from build123d import *

# Parameters (mm, degrees)
F0_W     = 12.7
F0_H     = 12.7
F0_R     = 2.54
F1_DEPTH = 6.35
F2_SIZE  = 2.54
F3_R     = 0.254


with BuildPart() as f1:
    # F0 (on Top) → F1 (new body)
    with BuildSketch(Plane.XY):
        Rectangle(F0_W, F0_H)
        Circle(F0_R, mode=Mode.SUBTRACT)
    extrude(amount=F1_DEPTH)

    # F2
    f2_edges = [f1.edges().sort_by_distance(p)[0] for p in [
        (-2.54, 0, 0),
    ]]
    chamfer(f2_edges, length=F2_SIZE)

    # F3
    f3_edges = [f1.edges().sort_by_distance(p)[0] for p in [
        (0, -6.35, 6.35),
        (0, -6.35, 0),
        (6.35, 0, 0),
        (6.35, 0, 6.35),
        (6.35, -6.35, 3.175),
        (6.35, 6.35, 3.175),
        (0, 6.35, 6.35),
        (-6.35, 6.35, 3.175),
        (-6.35, 0, 6.35),
        (-6.35, -6.35, 3.175),
        (-6.35, 0, 0),
        (0, 6.35, 0),
    ]]
    fillet(f3_edges, radius=F3_R)


solid = f1.part
Geometry check sheet. Reference: the model listing, model coordinates, mm. Round coordinates to 2 decimals unless told otherwise and drop trailing zeros. Order: outer loops, then holes, each group sorted by start corner. A loop starts at its lowest first (then second) coordinate and runs counter-clockwise, first axis right, second up. Notation, with made-up numbers: M 63.5,80 L 113.5,80 A10 ccw 113.5,87 Z; hole C -34,74 d6. An arc over 180 degrees is marked long. Answer in a Markdown table with one row per item.
(1) Sectioned sample at A-A, the plane x = 0. Record the cut outline in (y, z), and give its area (3 significant figures).
Responses:
| item | result |
|---|---|
| outline | M -6.35,0.25 A0.25 ccw -6.1,0 L -5.08,0 L -2.54,2.54 L -2.54,6.35 L -6.1,6.35 A0.25 ccw -6.35,6.1 Z; M 2.54,2.54 L 5.08,0 L 6.1,0 A0.25 ccw 6.35,0.25 L 6.35,6.1 A0.25 ccw 6.1,6.35 L 2.54,6.35 Z |
| area | 41.9 mm² |
(2) Sectioned sample at D-D, the plane z = 3.5. Record the cut outline in (x, y).
Responses:
| item | result |
|---|---|
| outline | M -6.35,-6.1 A0.25 ccw -6.1,-6.35 L 6.1,-6.35 A0.25 ccw 6.35,-6.1 L 6.35,6.1 A0.25 ccw 6.1,6.35 L -6.1,6.35 A0.25 ccw -6.35,6.1 Z; hole C 0,0 d5.08 |
(3) Sectioned sample at B-B, the plane z = 2. Record the cut outline in (x, y).
Responses:
| item | result |
|---|---|
| outline | M -6.35,-6.1 A0.25 ccw -6.1,-6.35 L 6.1,-6.35 A0.25 ccw 6.35,-6.1 L 6.35,6.1 A0.25 ccw 6.1,6.35 L -6.1,6.35 A0.25 ccw -6.35,6.1 Z; hole C 0,0 d6.16 |
(4) Scan lines: probe 1 along Y at (x, z) = (0, 5.15); probe 2 along X at (y, z) = (2, 2.5); probe 3 along X at (y, z) = (0.75, 1.5). Record each from-to range of solid material in increasing order. Write a range as from..to.
Responses:
| item | result |
|---|---|
| probe 1 | y = -6.35..-2.54, 2.54..6.35 |
| probe 2 | x = -6.35..-1.63, 1.63..6.35 |
| probe 3 | x = -6.35..-3.5, 3.5..6.35 |
(5) Draft check along X on faces 1 (the face through (1.245, -2.394, 2.381)), 2 (the face through (-0.33, 2.52, 4.42)), 3 (the face through (-3, 0, 6.35)), 4 (the face through (6.35, 0, 3)). Enter one of: released by +X, released by -X, zero draft, split by the parting line, or undercut.
Responses:
| item | result |
|---|---|
| face 1 | undercut |
| face 2 | undercut |
| face 3 | zero draft |
| face 4 | released by +X |
